Geometry check sheet. Reference: the model listing, model coordinates, mm. A direction names the side the tool comes from. Coordinates: 2 decimals unless noted, no trailing zeros. Loops run counter-clockwise (first coordinate to the right, second up) from the corner with the lowest first, then second, coordinate; pieces in that order, holes last. Notation, with made-up numbers: M 36.5,-19 L 66.5,-19 A18 ccw 66.5,3 Z; hole C -11,-7 d3. An arc over 180 degrees is marked long. One line per question, with ' | ' between items. Start each with the question number.
from build123d import *

# Parameters (mm, degrees)
SKETCH1_R           = 3
BOSS_EXTRUDE1_DEPTH = 2
SKETCH2_R           = 1.5
BOSS_EXTRUDE2_DEPTH = 15
SKETCH3_W           = 0.9
SKETCH3_H           = 0.9
SKETCH3_W_2         = 1.05
SKETCH3_H_2         = 1.05
CUT_EXTRUDE1_DEPTH  = 1.9
FILLET1_R           = 0.4


with BuildPart() as part:
    # Sketch1 → Boss-Extrude1 (new body)
    with BuildSketch(Plane(origin=(0, 0, 0), x_dir=(1, 0, 0), z_dir=(0, 1, 0))):
        Circle(SKETCH1_R)
    extrude(amount=BOSS_EXTRUDE1_DEPTH)

    # Sketch2 → Boss-Extrude2 (add)
    with BuildSketch(Plane(origin=(0, 2, 0), x_dir=(1, 0, 0), z_dir=(0, 1, 0))):
        Circle(SKETCH2_R)
    extrude(amount=BOSS_EXTRUDE2_DEPTH)

    # Sketch3 → Cut-Extrude1 (cut)
    with BuildSketch(Plane(origin=(0, 0, 0), x_dir=(-1, 0, 0), z_dir=(0, -1, 0))):
        Rectangle(SKETCH3_W, SKETCH3_H)
        with Locations((0.975, 0)):
            Rectangle(SKETCH3_W_2, SKETCH3_H)
        with Locations((0, -0.975)):
            Rectangle(SKETCH3_W, SKETCH3_H_2)
        with Locations((-0.975, 0)):
            Rectangle(SKETCH3_W_2, SKETCH3_H)
        with Locations((0, 0.975)):
            Rectangle(SKETCH3_W, SKETCH3_H_2)
    extrude(amount=-CUT_EXTRUDE1_DEPTH, mode=Mode.SUBTRACT)

    # Fillet1
    fillet1_edges = [part.edges().sort_by_distance(p)[0] for p in [
        (-3, 0, 0),
        (-3, 2, 0),
    ]]
    fillet(fillet1_edges, radius=FILLET1_R)


solid = part.part
1. Sectioned sample at A-A (z = 0). Record the cut outline in (x, y).
2. Depth check by flat-ended pin: pin 1 Ø1.2 at (x, y) = (-0.5, 1.5) entering from -Z; pin 2 Ø1.5 at (x, y) = (-2, 2.5) entering from +Z; pin 3 Ø0.5 at (y, z) = (1, -1) entering from -X; pin 4 Ø1.5 at (x, z) = (-2, -2.5) entering from +Y. Enter the tip coordinate at first touch or a pass-through.
3. Tool access check on faces 1 (the flat face through (-0.45, 1, 1)), 2 (the flat face through (0, 17, 0)), 3 (the cylindrical face through (-1.5, 9.4, -0.07)). Record the directions out of +Z, -Z, +X, -X, +Y, -Y that give a thin tool (end or side, any length) a straight path to the whole face; none if there is none.
4. Sectioned sample at C-C (y = 4.5). Record the cut outline in (x, z), and give its area (3 significant figures).
5. Sectioned sample at B-B (x = 0). Record the cut outline in (y, z).
6. Thickness scan on line 1 (Y direction, x = -2.3, z = 0.55); line 2 (X direction, y = 1.25, z = 1.2); line 3 (Z direction, x = -0.9, y = 6). Record the ranges inside material, lowest first.
7. Draft check along Z on faces 4 (the cylindrical face through (-3, 1, 0)), 5 (the flat face through (2, 2, 0)), 6 (the flat face through (-1, 1, -0.45)). Enter one of: +Z half, -Z half, draft (parallel to the pull), parting line (faces both ways), or undercut.
Result:
1) outline: M -3,0.4 A0.4 ccw -2.6,0 L -1.5,0 L -1.5,1.9 L 1.5,1.9 L 1.5,0 L 2.6,0 A0.4 ccw 3,0.4 L 3,1.6 A0.4 ccw 2.6,2 L 1.5,2 L 1.5,17 L -1.5,17 L -1.5,2 L -2.6,2 A0.4 ccw -3,1.6 Z
2) pin 1: stops at z = -3 | pin 2: stops at z = 2.42 | pin 3: stops at x = -2.9 | pin 4: stops at y = 2
3) face 1: -Y | face 2: +Z, -Z, +X, -X, +Y | face 3: +Y
4) outline: C 0,0 d3 | area: 7.07 mm2
5) outline: M 0,-2.6 A0.4 ccw 0.4,-3 L 1.6,-3 A0.4 ccw 2,-2.6 L 2,-1.5 L 17,-1.5 L 17,1.5 L 2,1.5 L 2,2.6 A0.4 ccw 1.6,3 L 0.4,3 A0.4 ccw 0,2.6 L 0,1.5 L 1.9,1.5 L 1.9,-1.5 L 0,-1.5 Z
6) line 1: y = 0 to 2 | line 2: x = -2.75 to -0.45, 0.45 to 2.75 | line 3: z = -1.2 to 1.2
7) face 4: parting line | face 5: draft | face 6: undercut
